```python
from build123d import *

# Parameters (mm, degrees)
SKETCH1_R                      = 60
BOSS_EXTRUDE1_DEPTH            = 6
CUT_EXTRUDE1_DEPTH             = 86.064681273
CUT_EXTRUDE1_DEPTH_BACK        = 86.064681273
SKETCH2_R                      = 13
F_4_0MM_DOWEL_HOLE1_D          = 5.6
F_1_0MM_DOWEL_HOLE1_D          = 5.6
CBORE_FOR_M2_SHCS3_D           = 2.4
CBORE_FOR_M2_SHCS3_CBORE_D     = 4.4
CBORE_FOR_M2_SHCS3_CBORE_DEPTH = 2


with BuildPart() as part:
    # Sketch1 → Boss-Extrude1 (new body)
    with BuildSketch(Plane.XY):
        Circle(SKETCH1_R)
    extrude(amount=-BOSS_EXTRUDE1_DEPTH)

    # Sketch2 → Cut-Extrude1 (cut, two sides: drawn at the far end of the back side and taken through both)
    with BuildSketch(Plane(origin=(0, 0, -6), x_dir=(-1, 0, 0), z_dir=(0, 0, -1)).offset(-CUT_EXTRUDE1_DEPTH_BACK)):
        Circle(SKETCH2_R)
    extrude(amount=CUT_EXTRUDE1_DEPTH + CUT_EXTRUDE1_DEPTH_BACK, mode=Mode.SUBTRACT)

    # Ø4.0mm Dowel Hole1 (through all)
    with Locations(Plane(origin=(0, 0, -6), x_dir=(-1, 0, 0), z_dir=(0, 0, -1))):
        with Locations((0, 0), (0, -33.25), (-28.795344676, -16.625), (-28.795344676, 16.625), (0, 33.25), (28.795344676, 16.625), (28.795344676, -16.625)):
            Hole(F_4_0MM_DOWEL_HOLE1_D / 2)

    # Ø1.0mm Dowel Hole1 (through all)
    with Locations(Plane.XY):
        with Locations((17.903184603, 28.018538168), (-17.903184603, -28.018538168)):
            Hole(F_1_0MM_DOWEL_HOLE1_D / 2)

    # CBORE for M2 SHCS3 (through all)
    with Locations(Plane(origin=(0, 0, -6), x_dir=(-1, 0, 0), z_dir=(0, 0, -1))):
        with Locations((-55.665534129, 12.261660172), (-30.691173604, 48.031779717), (12.261660172, 55.665534129), (55.665534129, -12.261660172), (30.691173604, -48.031779717), (-12.261660172, -55.665534129)):
            CounterBoreHole(CBORE_FOR_M2_SHCS3_D / 2, CBORE_FOR_M2_SHCS3_CBORE_D / 2, CBORE_FOR_M2_SHCS3_CBORE_DEPTH)


solid = part.part
```
Build history of the part. All positions in model axes, mm. A direction names the side the tool comes from. Round coordinates to 2 decimals unless told otherwise and drop trailing zeros. Write each loop counter-clockwise with the first axis right and the second up, starting at its lowest first coordinate (ties: lowest second). Pieces come first, ordered by that corner, then holes. Notation, with made-up numbers: (62.5, 19.25) -> (85.5, 19.25) arc R17 ccw to (85.5, 33.25) -> close; hole circle Ø4 at (2, -37). An arc over 180 degrees is marked (long way). Put each result on its own line as item: value.
Item 1: Slice it at A-A, the plane y = 0. Give the cut face in (x, z), plus the area to 3 significant figures.
Here are the results:
outline: (-60, -6) -> (-13, -6) -> (-13, 0) -> (-60, 0) -> close; (13, -6) -> (60, -6) -> (60, 0) -> (13, 0) -> close
area: 564 mm^2
Item 2: Two-plate mould, pull along Y, no slides. Class faces 1 (the face through (-1, 14, -6)), 2 (the face through (-59.94, 2.64, -2.96)), 3 (the face through (-12, 54, -4)): pulls with the +Y half, pulls with the -Y half, needs draft (parallel to the pull), parting line crosses it, or undercut.
Here are the results:
face 1: needs draft
face 2: parting line crosses it
face 3: undercut
Item 3: Tool access for faces 4 (the face through (28.66, 47.19, -5.01)), 5 (the face through (-1, 14, 0)): list every direction of +Z, -Z, +X, -X, +Y, -Y with a clear straight run to the whole face (end or side of a thin tool).
Here are the results:
face 4: -Z
face 5: +Z, +X, -X, +Y, -Y
Item 4: Flat gauge pins, fed straight in: P1, Ø2, axis at x = 12.5, y = -56.5, coming from the -Z side; P2, Ø4, axis at x = 12.26, y = -55.67, coming from the +Z side; P3, Ø1.5, axis at x = -4.5, z = -0.5, coming from the -Y side; P4, Ø3, axis at x = -34, z = -4.5, coming from the +Y side. Where does each tip first touch, or does it go through?
Here are the results:
P1: stops at z = -4
P2: stops at z = 0
P3: stops at y = -59.88
P4: stops at y = 50.44
Item 5: Slice it at D-D, the plane x = 16.5. Give the cut face in (y, z), plus the area to 3 significant figures.
Here are the results:
outline: (-57.69, -6) -> (25.6, -6) -> (25.6, 0) -> (-57.69, 0) -> close; (30.44, -6) -> (57.69, -6) -> (57.69, 0) -> (30.44, 0) -> close
area: 663 mm^2
Item 6: Slice it at C-C, the plane z = -2.6. Count the separate pieces of the cut face and the enclosed holes in it, plus the area to 3 significant figures.
Here are the results:
separate pieces: 1
enclosed holes: 15
area: 10,600 mm^2
Item 7: Slice it at B-B, the plane x = 0. Give the cut face in (y, z).
Here are the results:
outline: (-60, -6) -> (-36.05, -6) -> (-36.05, 0) -> (-60, 0) -> close; (-30.45, -6) -> (-13, -6) -> (-13, 0) -> (-30.45, 0) -> close; (13, -6) -> (30.45, -6) -> (30.45, 0) -> (13, 0) -> close; (36.05, -6) -> (60, -6) -> (60, 0) -> (36.05, 0) -> close
Item 8: Wall check: probe 1 along Y at (x, z) = (0, -3.5); probe 2 along Y at (x, z) = (-27.5, -1.95); probe 3 along X at (y, z) = (-16.5, -5.45). Give the ranges that are in metal, low to high. Write a range as from..to.
Here are the results:
probe 1: y = -60..-36.05, -30.45..-13, 13..30.45, 36.05..60
probe 2: y = -53.33..-19.11, -14.14..14.14, 19.11..53.33
probe 3: x = -57.69..-31.59, -26..26, 31.59..57.69
